from build123d import *

# Parameters (mm, degrees)
SM_BASE_FLANGE_1_DEPTH = 910
SKETCH_6_W             = 101
SKETCH_6_H             = 30
CUT_EXTRUDE_1_DEPTH    = 37
SKETCH_7_W             = 17
SKETCH_7_H             = 97
CUT_EXTRUDE_2_DEPTH    = 24
SKETCH_8_R             = 6.5
SKETCH_8_R_2           = 3.25
CUT_EXTRUDE_3_DEPTH    = 10
SKETCH_9_R             = 3.25
CUT_EXTRUDE_4_DEPTH    = 10
CUT_EXTRUDE_7_DEPTH    = 10
CUT_EXTRUDE_8_DEPTH    = 10
SKETCH_16_R            = 3.25
SKETCH_16_R_2          = 6.5
CUT_EXTRUDE_9_DEPTH    = 10
SKETCH_17_R            = 2.5
CUT_EXTRUDE_10_DEPTH   = 10
SKETCH_25_R            = 4
SKETCH_25_R_2          = 2.5
CUT_EXTRUDE_16_DEPTH   = 10
SKETCH_26_R            = 3.25
CUT_EXTRUDE_17_DEPTH   = 10


# Sheet-metal steps are written as plain solids
with BuildPart() as part:
    # Sketch 1 → Базовая кромка1 (new, symmetric)
    with BuildSketch(Plane.XY):
        with BuildLine():
            Line((0, 0), (-31, 0))
            ThreePointArc((-31, 0), (-32.414213562, -0.585786438), (-33, -2))
            Line((-33, -2), (-33, -24))
            ThreePointArc((-33, -24), (-34.171572875, -26.828427125), (-37, -28))
            Line((-37, -28), (-179, -28))
            ThreePointArc((-179, -28), (-181.828427125, -26.828427125), (-183, -24))
            Line((-183, -24), (-183, 33))
            ThreePointArc((-183, 33), (-181.828427125, 35.828427125), (-179, 37))
            Line((-179, 37), (-170, 37))
            ThreePointArc((-170, 37), (-168.585786438, 37.585786438), (-168, 39))
            Line((-168, 39), (-168, 57))
            Line((-168, 57), (-166, 57))
            Line((-166, 57), (-166, 39))
            ThreePointArc((-166, 39), (-167.171572875, 36.171572875), (-170, 35))
            Line((-170, 35), (-179, 35))
            ThreePointArc((-179, 35), (-180.414213562, 34.414213562), (-181, 33))
            Line((-181, 33), (-181, -24))
            ThreePointArc((-181, -24), (-180.414213562, -25.414213562), (-179, -26))
            Line((-179, -26), (-37, -26))
            ThreePointArc((-37, -26), (-35.585786438, -25.414213562), (-35, -24))
            Line((-35, -24), (-35, -2))
            ThreePointArc((-35, -2), (-33.828427125, 0.828427125), (-31, 2))
            Line((-31, 2), (0, 2))
            Line((0, 2), (0, 0))
        make_face()
    extrude(amount=SM_BASE_FLANGE_1_DEPTH, both=True)

    # Эскиз6 → Cut-Extrude 1 (cut)
    with BuildSketch(Plane(origin=(0, 0, 0), x_dir=(0, 0, -1), z_dir=(1, 0, 0))):
        with Locations((-859.5, -13)):
            Rectangle(SKETCH_6_W, SKETCH_6_H)
        with Locations((859.5, -13)):
            Rectangle(SKETCH_6_W, SKETCH_6_H)
    extrude(amount=-CUT_EXTRUDE_1_DEPTH, mode=Mode.SUBTRACT)

    # Эскиз7 → Вырез-Вытянуть2 (cut)
    with BuildSketch(Plane(origin=(0, 57, 0), x_dir=(1, 0, 0), z_dir=(0, 1, 0))):
        with Locations((-174.5, -861.5)):
            Rectangle(SKETCH_7_W, SKETCH_7_H)
        with Locations((-174.5, 861.5)):
            Rectangle(SKETCH_7_W, SKETCH_7_H)
    extrude(amount=-CUT_EXTRUDE_2_DEPTH, mode=Mode.SUBTRACT)

    # Эскиз8 → Вырез-Вытянуть3 (cut)
    with BuildSketch(Plane(origin=(0, -26, 0), x_dir=(1, 0, 0), z_dir=(0, 1, 0))):
        with Locations(Location((-108, 860, 0), (0, 0, 180))):
            Circle(SKETCH_8_R)
        with Locations(Location((-68, 890, 0), (0, 0, 180))):
            Circle(SKETCH_8_R_2)
        with Locations(Location((-148, 890, 0), (0, 0, 180))):
            Circle(SKETCH_8_R_2)
        with Locations(Location((-148, 840, 0), (0, 0, 180))):
            Circle(SKETCH_8_R_2)
        with Locations(Location((-68, 840, 0), (0, 0, 180))):
            Circle(SKETCH_8_R_2)
        with Locations(Location((-148, 770, 0), (0, 0, 180))):
            Circle(SKETCH_8_R_2)
        with Locations((-148, -770)):
            Circle(SKETCH_8_R_2)
        with Locations((-148, -890)):
            Circle(SKETCH_8_R_2)
        with Locations((-148, -840)):
            Circle(SKETCH_8_R_2)
        with Locations((-68, -840)):
            Circle(SKETCH_8_R_2)
        with Locations((-68, -890)):
            Circle(SKETCH_8_R_2)
    extrude(amount=-CUT_EXTRUDE_3_DEPTH, mode=Mode.SUBTRACT)

    # Эскиз9 → Вырез-Вытянуть4 (cut)
    with BuildSketch(Plane(origin=(0, -26, 0), x_dir=(1, 0, 0), z_dir=(0, 1, 0))):
        with Locations(Location((-68, -190, 0), (0, 0, 180))):
            Circle(SKETCH_9_R)
        with Locations(Location((-148, -190, 0), (0, 0, 180))):
            Circle(SKETCH_9_R)
        with Locations(Location((-148, -210, 0), (0, 0, 180))):
            Circle(SKETCH_9_R)
        with Locations(Location((-68, -210, 0), (0, 0, 180))):
            Circle(SKETCH_9_R)
    cut_extrude_4 = extrude(amount=-CUT_EXTRUDE_4_DEPTH, mode=Mode.SUBTRACT)

    # Зеркальное отражение1: Вырез-Вытянуть4 across plane
    add(cut_extrude_4.mirror(Plane(origin=(-77.5, 77.5, 0), x_dir=(0, 0, 1), z_dir=(-0.7071067811865476, 0.7071067811865475, 0))), mode=Mode.SUBTRACT)

    # Эскиз14 → Вырез-Вытянуть7 (cut)
    with BuildSketch(Plane.XZ):
        with BuildLine():
            Line((-12, 566.25), (-7, 566.25))
            ThreePointArc((-7, 566.25), (-3.75, 563), (-7, 559.75))
            Line((-7, 559.75), (-12, 559.75))
            ThreePointArc((-12, 559.75), (-15.25, 563), (-12, 566.25))
        make_face()
        with BuildLine():
            Line((-12, 541.25), (-7, 541.25))
            ThreePointArc((-7, 541.25), (-3.75, 538), (-7, 534.75))
            Line((-7, 534.75), (-12, 534.75))
            ThreePointArc((-12, 534.75), (-15.25, 538), (-12, 541.25))
        make_face()
        with BuildLine():
            Line((-12, -626.75), (-7, -626.75))
            ThreePointArc((-7, -626.75), (-3.75, -630), (-7, -633.25))
            Line((-7, -633.25), (-12, -633.25))
            ThreePointArc((-12, -633.25), (-15.25, -630), (-12, -626.75))
        make_face()
        with BuildLine():
            Line((-12, -651.75), (-7, -651.75))
            ThreePointArc((-7, -651.75), (-3.75, -655), (-7, -658.25))
            Line((-7, -658.25), (-12, -658.25))
            ThreePointArc((-12, -658.25), (-15.25, -655), (-12, -651.75))
        make_face()
    extrude(amount=-CUT_EXTRUDE_7_DEPTH, mode=Mode.SUBTRACT)

    # Эскиз15 → Вырез-Вытянуть8 (cut)
    with BuildSketch(Plane.ZY.offset(183)):
        with BuildLine():
            Line((-734.5, 5.5), (-705.5, 5.5))
            ThreePointArc((-705.5, 5.5), (-700, 0), (-705.5, -5.5))
            Line((-705.5, -5.5), (-734.5, -5.5))
            ThreePointArc((-734.5, -5.5), (-740, 0), (-734.5, 5.5))
        make_face()
        with BuildLine():
            Line((-85.5, -5.5), (-114.5, -5.5))
            ThreePointArc((-114.5, -5.5), (-120, 0), (-114.5, 5.5))
            Line((-114.5, 5.5), (-85.5, 5.5))
            ThreePointArc((-85.5, 5.5), (-80, 0), (-85.5, -5.5))
        make_face()
        with BuildLine():
            Line((14.5, -5.5), (-14.5, -5.5))
            ThreePointArc((-14.5, -5.5), (-20, 0), (-14.5, 5.5))
            Line((-14.5, 5.5), (14.5, 5.5))
            ThreePointArc((14.5, 5.5), (20, 0), (14.5, -5.5))
        make_face()
        with BuildLine():
            Line((114.5, -5.5), (85.5, -5.5))
            ThreePointArc((85.5, -5.5), (80, 0), (85.5, 5.5))
            Line((85.5, 5.5), (114.5, 5.5))
            ThreePointArc((114.5, 5.5), (120, 0), (114.5, -5.5))
        make_face()
        with BuildLine():
            Line((734.5, -5.5), (705.5, -5.5))
            ThreePointArc((705.5, -5.5), (700, 0), (705.5, 5.5))
            Line((705.5, 5.5), (734.5, 5.5))
            ThreePointArc((734.5, 5.5), (740, 0), (734.5, -5.5))
        make_face()
    extrude(amount=-CUT_EXTRUDE_8_DEPTH, mode=Mode.SUBTRACT)

    # Эскиз16 → Вырез-Вытянуть9 (cut)
    with BuildSketch(Plane.ZY.offset(183)):
        with Locations((890, 7)):
            Circle(SKETCH_16_R)
        with Locations((860, 7)):
            Circle(SKETCH_16_R_2)
        with Locations((840, 7)):
            Circle(SKETCH_16_R)
        with Locations((770, 7)):
            Circle(SKETCH_16_R)
        with Locations(Location((-770, 7, 0), (0, 0, 180))):
            Circle(SKETCH_16_R)
        with Locations(Location((-840, 7, 0), (0, 0, 180))):
            Circle(SKETCH_16_R)
        with Locations(Location((-860, 7, 0), (0, 0, 180))):
            Circle(SKETCH_16_R_2)
        with Locations(Location((-890, 7, 0), (0, 0, 180))):
            Circle(SKETCH_16_R)
    extrude(amount=-CUT_EXTRUDE_9_DEPTH, mode=Mode.SUBTRACT)

    # Эскиз17 → Вырез-Вытянуть10 (cut)
    with BuildSketch(Plane.ZY.offset(168)):
        with Locations((775, 47)):
            Circle(SKETCH_17_R)
        with Locations((-500, 47)):
            Circle(SKETCH_17_R)
        with Locations((-775, 47)):
            Circle(SKETCH_17_R)
        with Locations((-797, 50)):
            Circle(SKETCH_17_R)
        with Locations((797, 50)):
            Circle(SKETCH_17_R)
        with Locations((-750, 47)):
            Circle(SKETCH_17_R)
        with Locations((-725, 47)):
            Circle(SKETCH_17_R)
        with Locations((-700, 47)):
            Circle(SKETCH_17_R)
        with Locations((-450, 47)):
            Circle(SKETCH_17_R)
        with Locations((-400, 47)):
            Circle(SKETCH_17_R)
        with Locations((-350, 47)):
            Circle(SKETCH_17_R)
        with Locations((-300, 47)):
            Circle(SKETCH_17_R)
        with Locations((-250, 47)):
            Circle(SKETCH_17_R)
        with Locations((-200, 47)):
            Circle(SKETCH_17_R)
        with Locations((-150, 47)):
            Circle(SKETCH_17_R)
        with Locations((-100, 47)):
            Circle(SKETCH_17_R)
        with Locations((-50, 47)):
            Circle(SKETCH_17_R)
        with Locations((0, 47)):
            Circle(SKETCH_17_R)
        with Locations((50, 47)):
            Circle(SKETCH_17_R)
        with Locations((100, 47)):
            Circle(SKETCH_17_R)
        with Locations((150, 47)):
            Circle(SKETCH_17_R)
        with Locations((200, 47)):
            Circle(SKETCH_17_R)
        with Locations((250, 47)):
            Circle(SKETCH_17_R)
        with Locations((300, 47)):
            Circle(SKETCH_17_R)
        with Locations((350, 47)):
            Circle(SKETCH_17_R)
        with Locations((750, 47)):
            Circle(SKETCH_17_R)
        with Locations((725, 47)):
            Circle(SKETCH_17_R)
        with Locations((700, 47)):
            Circle(SKETCH_17_R)
        with Locations((400, 47)):
            Circle(SKETCH_17_R)
        with Locations((450, 47)):
            Circle(SKETCH_17_R)
        with Locations((500, 47)):
            Circle(SKETCH_17_R)
        with Locations((550, 47)):
            Circle(SKETCH_17_R)
        with Locations((600, 47)):
            Circle(SKETCH_17_R)
        with Locations((650, 47)):
            Circle(SKETCH_17_R)
    extrude(amount=-CUT_EXTRUDE_10_DEPTH, mode=Mode.SUBTRACT)

    # Эскиз25 → Вырез-Вытянуть16 (cut)
    with BuildSketch(Plane.XZ):
        with Locations(Location((-16, -755, 0), (0, 0, 270))):
            Circle(SKETCH_25_R)
        with Locations(Location((-16, 0, 0), (0, 0, 270))):
            Circle(SKETCH_25_R)
        with Locations(Location((-20, 772.5, 0), (0, 0, 270))):
            Circle(SKETCH_25_R_2)
        with Locations(Location((-20, 747.5, 0), (0, 0, 270))):
            Circle(SKETCH_25_R_2)
    extrude(amount=-CUT_EXTRUDE_16_DEPTH, mode=Mode.SUBTRACT)

    # Эскиз26 → Вырез-Вытянуть17 (cut)
    with BuildSketch(Plane.XZ):
        with Locations(Location((-10, -797, 0), (0, 0, 270))):
            Circle(SKETCH_26_R)
        with Locations(Location((-10, 797, 0), (0, 0, 270))):
            Circle(SKETCH_26_R)
    extrude(amount=-CUT_EXTRUDE_17_DEPTH, mode=Mode.SUBTRACT)


solid = part.part
Read the model definition and answer for the solid it produces. Units are mm, in the model's axes. A direction names the side the tool comes from. Round coordinates to 2 decimals unless told otherwise and drop trailing zeros. Write each loop counter-clockwise with the first axis right and the second up, starting at its lowest first coordinate (ties: lowest second). Pieces come first, ordered by that corner, then holes.
1. Which of the six approach directions +Z, -Z, +X, -X, +Y, -Y give full straight-line access (tool end or side, diameter ignored) to faces 1 (the face through (-26.6, 0.3, -809)), 2 (the face through (-15, 0, 11)), 3 (the face through (-26.6, 0.3, 809)), 4 (the face through (-16, 2, 11))?
2. Straight lines are drawn through the part: L1, parallel to X at y = -6, z = 142; L2, parallel to X at y = 50.5, z = 251.5; L3, parallel to X at y = 18.5, z = -609.5. For each, find the intervals that lie inside material, in ascending order.
3. The part is cut by section A-A, the plane z = 331.5. Determine the outline of the cut face in (x, y).
4. Given pin 1 Ø3 at (y, z) = (47, -775) entering from -X; pin 2 Ø6.5 at (y, z) = (47, -100) entering from -X; pin 3 Ø6.5 at (y, z) = (47, -200) entering from +X; pin 4 Ø1.5 at (y, z) = (10, -359) entering from +X, each flat-ended and moving along its own axis, determine where each tip first touches the part or whether it passes through.
5. Determine the mould class of faces 5 (the face through (-110, -27, -910)), 6 (the face through (-181, 11, 13)), 7 (the face through (-107, -28, 13)) for opening direction Y: pulls with the +Y half, pulls with the -Y half, needs draft (parallel to the pull), parting line crosses it, or undercut.
Values:
1. face 1: -Z, +X, +Y, -Y
1. face 2: +Z, -Z, +X, -Y
1. face 3: +Z, +X, +Y, -Y
1. face 4: +Z, -Z, +X, +Y
2. L1: x = -183 to -181, -35 to -33
2. L2: x = -168 to -166
2. L3: x = -183 to -181
3. outline: (-183, -24) arc R4 ccw to (-179, -28) - (-37, -28) arc R4 ccw to (-33, -24) - (-33, -2) arc R2 cw to (-31, 0) - (0, 0) - (0, 2) - (-31, 2) arc R4 ccw to (-35, -2) - (-35, -24) arc R2 cw to (-37, -26) - (-179, -26) arc R2 cw to (-181, -24) - (-181, 33) arc R2 cw to (-179, 35) - (-170, 35) arc R4 ccw to (-166, 39) - (-166, 57) - (-168, 57) - (-168, 39) arc R2 cw to (-170, 37) - (-179, 37) arc R4 ccw to (-183, 33) - close
4. pin 1: passes through
4. pin 2: stops at x = -168
4. pin 3: stops at x = -166
4. pin 4: stops at x = -181
5. face 5: needs draft
5. face 6: undercut
5. face 7: pulls with the -Y half
